Geometry: final body of the model. Coordinates: model frame, mm. Give positions to 0.01 mm unless a question says otherwise; leave off trailing zeros. Loops run counter-clockwise (first coordinate to the right, second up) from the corner with the lowest first, then second, coordinate; pieces in that order, holes last. Notation, with made-up numbers: (19, 71.5) - (47, 71.5) arc R27 ccw to (47, 96.5) - close; hole circle Ø3 at (-23, 68). An arc over 180 degrees is marked (long way). Answer in a Markdown table with one row per item.
from build123d import *

# Parameters (mm, degrees)
SKETCH_2_W      = 95
SKETCH_2_H      = 105
SKETCH_2_R      = 2.1
SKETCH_2_R_2    = 13.25
SKETCH_2_R_3    = 1.6
EXTRUDE_1_DEPTH = 3
FILLET_1_R      = 5
CHAMFER_1_SIZE  = 1.5


with BuildPart() as part:
    # ｽｹｯﾁ2 → ﾎﾞｽ - 押し出し1 (new body)
    with BuildSketch(Plane.XY):
        with Locations((16.5, 0)):
            Rectangle(SKETCH_2_W, SKETCH_2_H)
        with Locations((-13, -17.5)):
            Circle(SKETCH_2_R, mode=Mode.SUBTRACT)
        with Locations((-13, -43.5)):
            Circle(SKETCH_2_R, mode=Mode.SUBTRACT)
        with Locations((13, -17.5)):
            Circle(SKETCH_2_R, mode=Mode.SUBTRACT)
        with Locations((13, -43.5)):
            Circle(SKETCH_2_R, mode=Mode.SUBTRACT)
        with Locations((41, 0)):
            Circle(SKETCH_2_R_2, mode=Mode.SUBTRACT)
        with Locations((53.374368671, 12.374368671)):
            Circle(SKETCH_2_R, mode=Mode.SUBTRACT)
        with Locations((28.625631329, -12.374368671)):
            Circle(SKETCH_2_R, mode=Mode.SUBTRACT)
        with Locations((53.374368671, -12.374368671)):
            Circle(SKETCH_2_R, mode=Mode.SUBTRACT)
        with Locations((28.625631329, 12.374368671)):
            Circle(SKETCH_2_R, mode=Mode.SUBTRACT)
        with Locations((-23.5, 45)):
            Circle(SKETCH_2_R_3, mode=Mode.SUBTRACT)
        with Locations((-23.5, -45)):
            Circle(SKETCH_2_R_3, mode=Mode.SUBTRACT)
        with Locations((56.5, -45)):
            Circle(SKETCH_2_R_3, mode=Mode.SUBTRACT)
        with Locations((56.5, 45)):
            Circle(SKETCH_2_R_3, mode=Mode.SUBTRACT)
        with Locations((-13, 17.5)):
            Circle(SKETCH_2_R, mode=Mode.SUBTRACT)
        with Locations((13, 17.5)):
            Circle(SKETCH_2_R, mode=Mode.SUBTRACT)
        with Locations((13, 43.5)):
            Circle(SKETCH_2_R, mode=Mode.SUBTRACT)
        with Locations((-13, 43.5)):
            Circle(SKETCH_2_R, mode=Mode.SUBTRACT)
    extrude(amount=EXTRUDE_1_DEPTH)

    # ﾌｨﾚｯﾄ1
    fillet_1_edges = [part.edges().sort_by_distance(p)[0] for p in [
        (64, -52.5, 1.5),
        (-31, -52.5, 1.5),
        (-31, 52.5, 1.5),
        (64, 52.5, 1.5),
    ]]
    fillet(fillet_1_edges, radius=FILLET_1_R)

    # 面取り1
    chamfer_1_edges = [part.edges().sort_by_distance(p)[0] for p in [
        (-15.1, -17.5, 3),
        (-15.1, -43.5, 3),
        (10.9, -17.5, 3),
        (10.9, -43.5, 3),
        (-15.1, 17.5, 3),
        (10.9, 17.5, 3),
        (10.9, 43.5, 3),
        (-15.1, 43.5, 3),
    ]]
    chamfer(chamfer_1_edges, length=CHAMFER_1_SIZE)


solid = part.part
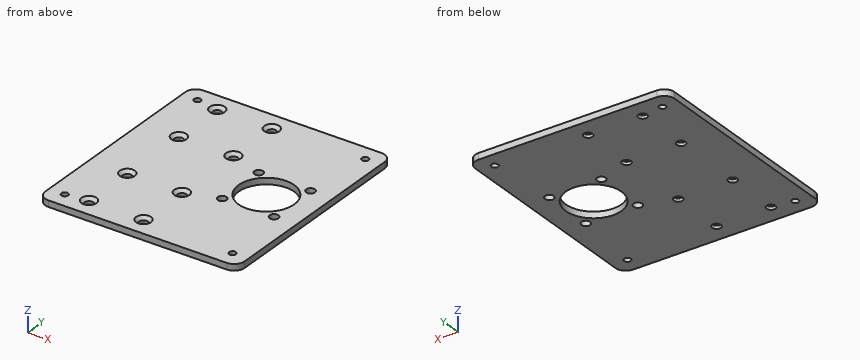
Q1. Cut plane D-D (y = 0). Output: boundary loops of the cut face in (x, z), and give its area (4 significant figures).
Check values:
| item | result |
|---|---|
| outline | (-31, 0) - (27.75, 0) - (27.75, 3) - (-31, 3) - close; (54.25, 0) - (64, 0) - (64, 3) - (54.25, 3) - close |
| area | 205.5 mm² |
Q2. Cut plane B-B (x = 41). Output: boundary loops of the cut face in (y, z), and give its area (4 significant figures).
Check values:
| item | result |
|---|---|
| outline | (-52.5, 0) - (-13.25, 0) - (-13.25, 3) - (-52.5, 3) - close; (13.25, 0) - (52.5, 0) - (52.5, 3) - (13.25, 3) - close |
| area | 235.5 mm² |
Q3. First-contact query: pin 1 (4 mm diameter, centred on x = 28.63, y = 12.37, fed in from -Z); pin 2 (5 mm diameter, centred on x = 13, y = 43.5, fed in from +Z); pin 3 (5.5 mm diameter, centred on x = -13, y = -17.5, fed in from +Z); pin 4 (6.5 mm diameter, centred on x = 13, y = -17.5, fed in from +Z). Flat tips, straight axial feed; report the tip coordinate or a pass-through.
Check values:
| item | result |
|---|---|
| pin 1 | through |
| pin 2 | z = 1.9 |
| pin 3 | z = 2.15 |
| pin 4 | z = 2.65 |
Q4. Cut plane A-A (x = -23.5). Output: boundary loops of the cut face in (y, z), and give its area (3 significant figures).
Check values:
| item | result |
|---|---|
| outline | (-52.5, 0) - (-46.6, 0) - (-46.6, 3) - (-52.5, 3) - close; (-43.4, 0) - (43.4, 0) - (43.4, 3) - (-43.4, 3) - close; (46.6, 0) - (52.5, 0) - (52.5, 3) - (46.6, 3) - close |
| area | 296 mm² |
Q5. Cut plane C-C (y = 17.5). Output: boundary loops of the cut face in (x, z).
Check values:
| item | result |
|---|---|
| outline | (-31, 0) - (-15.1, 0) - (-15.1, 1.5) - (-16.6, 3) - (-31, 3) - close; (-10.9, 0) - (10.9, 0) - (10.9, 1.5) - (9.4, 3) - (-9.4, 3) - (-10.9, 1.5) - close; (15.1, 0) - (64, 0) - (64, 3) - (16.6, 3) - (15.1, 1.5) - close |
Q6. Material intervals for line 1 along Y through (x, z) = (13, 0.4); line 2 along Y through (x, z) = (-23.5, 1.1); line 3 along Y through (x, z) = (41, 2), sorted ascending.
Check values:
| item | result |
|---|---|
| line 1 | -52.5 to -45.6, -41.4 to -19.6, -15.4 to 15.4, 19.6 to 41.4, 45.6 to 52.5 |
| line 2 | -52.5 to -46.6, -43.4 to 43.4, 46.6 to 52.5 |
| line 3 | -52.5 to -13.25, 13.25 to 52.5 |
